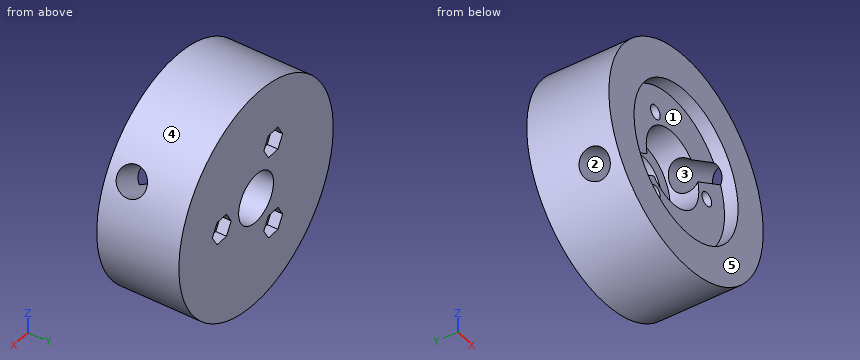
```python
from build123d import *

# Parameters (mm, degrees)
TYRE_SEAT_BLANK_SKETCH_R        = 27
TYRE_SEAT_BLANK_DEPTH           = 20
AXLE_CLEARANCE_SKETCH_R         = 6.1
AXLE_CLEARANCE_DEPTH            = 20.2
HUB_NECK_SOCKET_SKETCH_R        = 9.2
HUB_NECK_SOCKET_DEPTH           = 10.5
HUB_FLANGE_SOCKET_SKETCH_R      = 18.2
HUB_FLANGE_SOCKET_DEPTH         = 3.5
RIM_BOLT_PATTERN_SKETCH_R       = 1.7
RIM_BOLT_PATTERN_DEPTH          = 20.2
RIM_NUT_POCKETS_DEPTH           = 2.7
HUB_PIN_SERVICE_WINDOW_SKETCH_R = 3.6
HUB_PIN_SERVICE_WINDOW_DEPTH    = 56


with BuildPart() as part:
    # Tyre seat blank sketch → Tyre seat blank (new body)
    with BuildSketch(Plane(origin=(0, -283, 0), x_dir=(1, 0, 0), z_dir=(0, 1, 0))):
        with Locations(Location((-19.009182883, 53.244882879, 0), (0, 0, 270))):
            Circle(TYRE_SEAT_BLANK_SKETCH_R)
    extrude(amount=TYRE_SEAT_BLANK_DEPTH)

    # Axle clearance sketch → Axle clearance (cut)
    with BuildSketch(Plane(origin=(0, -283.1, 0), x_dir=(1, 0, 0), z_dir=(0, 1, 0))):
        with Locations(Location((-19.009182883, 53.244882879, 0), (0, 0, 270))):
            Circle(AXLE_CLEARANCE_SKETCH_R)
    extrude(amount=AXLE_CLEARANCE_DEPTH, mode=Mode.SUBTRACT)

    # Hub neck socket sketch → Hub neck socket (cut)
    with BuildSketch(Plane(origin=(0, -273.3, 0), x_dir=(1, 0, 0), z_dir=(0, 1, 0))):
        with Locations(Location((-19.009182883, 53.244882879, 0), (0, 0, 90))):
            Circle(HUB_NECK_SOCKET_SKETCH_R)
    extrude(amount=HUB_NECK_SOCKET_DEPTH, mode=Mode.SUBTRACT)

    # Hub flange socket sketch → Hub flange socket (cut)
    with BuildSketch(Plane(origin=(0, -266.3, 0), x_dir=(1, 0, 0), z_dir=(0, 1, 0))):
        with Locations(Location((-19.009182883, 53.244882879, 0), (0, 0, 270))):
            Circle(HUB_FLANGE_SOCKET_SKETCH_R)
    extrude(amount=HUB_FLANGE_SOCKET_DEPTH, mode=Mode.SUBTRACT)

    # Rim bolt pattern sketch → Rim bolt pattern (cut)
    with BuildSketch(Plane(origin=(0, -283.1, 0), x_dir=(1, 0, 0), z_dir=(0, 1, 0))):
        with Locations(Location((-7.009182883, 53.244882879, 0), (0, 0, 270))):
            Circle(RIM_BOLT_PATTERN_SKETCH_R)
        with Locations(Location((-25.009182883, 42.852578033, 0), (0, 0, 270))):
            Circle(RIM_BOLT_PATTERN_SKETCH_R)
        with Locations(Location((-25.009182883, 63.637187724, 0), (0, 0, 270))):
            Circle(RIM_BOLT_PATTERN_SKETCH_R)
    extrude(amount=RIM_BOLT_PATTERN_DEPTH, mode=Mode.SUBTRACT)

    # Rim nut pockets sketch → Rim nut pockets (cut)
    with BuildSketch(Plane(origin=(0, -283.1, 0), x_dir=(1, 0, 0), z_dir=(0, 1, 0))):
        Polygon((-3.709182883, 53.244882879), (-5.359182883, 56.102766711), (-8.659182883, 56.102766711), (-10.309182883, 53.244882879), (-8.659182883, 50.386999046), (-5.359182883, 50.386999046), align=None)
        Polygon((-21.709182883, 42.852578033), (-23.359182883, 45.710461866), (-26.659182883, 45.710461866), (-28.309182883, 42.852578033), (-26.659182883, 39.994694201), (-23.359182883, 39.994694201), align=None)
        Polygon((-21.709182883, 63.637187724), (-23.359182883, 66.495071557), (-26.659182883, 66.495071557), (-28.309182883, 63.637187724), (-26.659182883, 60.779303892), (-23.359182883, 60.779303892), align=None)
    extrude(amount=RIM_NUT_POCKETS_DEPTH, mode=Mode.SUBTRACT)

    # Hub pin service window sketch → Hub pin service window (cut)
    with BuildSketch(Plane(origin=(-61.561309066, 0, -35.542438361), x_dir=(0.4999999999999994, 0, -0.866025403784439), z_dir=(0.866025403784439, 0, 0.4999999999999994))):
        with Locations(Location((36.606829753, -269, 0), (0, 0, 180))):
            Circle(HUB_PIN_SERVICE_WINDOW_SKETCH_R)
    extrude(amount=HUB_PIN_SERVICE_WINDOW_DEPTH, mode=Mode.SUBTRACT)


with BuildPart() as body_2:
    # Mirror1: mirrored copy
    add(part.part.mirror(Plane(origin=(0, 0, 0), x_dir=(0, 0, 1), z_dir=(0, -1, 0))))


solid = body_2.part
```
Geometry: final body of the model. Coordinates: model frame, mm. Face numbers are marked on the shaded views. A direction names the side the tool comes from. Round coordinates to 2 decimals unless told otherwise and drop trailing zeros. Loops run counter-clockwise (first coordinate to the right, second up) from the corner with the lowest first, then second, coordinate; pieces in that order, holes last. Notation, with made-up numbers: (28, -29) -> (53, -29) arc R14 cw to (53, -12) -> close; hole circle Ø10 at (78.25, -32). An arc over 180 degrees is marked (long way). Use one line per item in the form item = value.
Item 1: Material intervals for probe 1 along Z at (x, y) = (-19, 268); probe 2 along Z at (x, y) = (-7, 269.75); probe 3 along Z at (x, y) = (-23.5, 277.5), sorted ascending.
Evaluation:
probe_1 = -80.24 to -62.44, -44.04 to -26.24
probe_2 = -77.43 to -54.94, -51.54 to -50.38, -42.25 to -29.06
probe_3 = -79.87 to -64.42, -62.85 to -57.37, -49.12 to -43.64, -42.07 to -26.62
Item 2: Draft query along X for the marked faces 3, 4 and 5. Return one class per face: released by +X, released by -X, zero draft, split by the parting line, or undercut.
Evaluation:
face_3 = undercut
face_4 = split by the parting line
face_5 = zero draft
Item 3: Cut plane B-B on y = 278.75. Output: boundary loops of the cut face in (x, z), then the cut area to 3 significant figures.
Evaluation:
outline = circle Ø54 at (-19.01, -53.24); hole circle Ø3.4 at (-25.01, -63.64); hole circle Ø3.4 at (-25.01, -42.85); hole circle Ø12.2 at (-19.01, -53.24); hole circle Ø3.4 at (-7.01, -53.24)
area = 2,150 mm2
Item 4: Contact query for flat-ended pins moving along their axis: pin 1 Ø1.5 at (x, y) = (-3.5, 271) entering from +Z; pin 2 Ø0.8 at (x, y) = (-25, 281.5) entering from -Z; pin 3 Ø1.5 at (x, y) = (-16, 267.5) entering from +Z. Output: stop coordinate, or through.
Evaluation:
pin_1 = -30.64
pin_2 = -79.66
pin_3 = -26.34
Item 5: Access query for the marked faces 1 and 2. Directions: +Z, -Z, +X, -X, +Y, -Y. A direction counts if a zero-diameter tool reaches every point of the face in a straight line with its end or side. Return the directions, or none.
Evaluation:
face_1 = -Y
face_2 = none
Item 6: Cut plane C-C on z = -75. Output: boundary loops of the cut face in (x, y), then the cut area to 3 significant figures.
Evaluation:
outline = (-35, 263) -> (-3.02, 263) -> (-3.02, 283) -> (-35, 283) -> close
area = 640 mm2
Item 7: Cut plane A-A on z = -36. Output: boundary loops of the cut face in (x, y).
Evaluation:
outline = (-39.78, 263) -> (-24.83, 263) -> (-24.83, 266.3) -> (-13.19, 266.3) -> (-13.19, 263) -> (1.77, 263) -> (1.77, 283) -> (-39.78, 283) -> close
